Part model, mm, in its own coordinate system. Face numbers are marked on the shaded views. A direction names the side the tool comes from. Coordinates: 2 decimals unless noted, no trailing zeros. Loops run counter-clockwise (first coordinate to the right, second up) from the corner with the lowest first, then second, coordinate; pieces in that order, holes last. Notation, with made-up numbers: M 53.5,-14 L 108.5,-14 A20 cw 108.5,-10 Z; hole C 65,-33 d10. An arc over 180 degrees is marked long. Answer as a JSON object with one key per item and string values. Group by question number.
1. Mould opens along Z. For the marked faces 1, 2 and 3 say: released by +Z, released by -Z, zero draft, split by the parting line, or undercut.
2. Saw through at A-A on y = 0.3. Write the cut outline in (x, z) (3 decimals), then the cut area to 3 significant figures.
3. Drill centre lines: L1, parallel to Z at x = -1.25, y = 1.1 (3 decimals); L2, parallel to X at y = 0.4, z = 0.5 (3 decimals); L3, parallel to Z at x = -1.25, y = 3.05. Where is each one in solid material? Low to high.
4. Drop flat-ended pins along their axis: pin 1 Ø4 at (x, z) = (-4, -3) entering from -Y; pin 2 Ø0.6 at (x, y) = (-0.5, 0.5) entering from +Z. Give the stop position or say it passes through.
5. Saw through at B-B on x = -4. Write the cut outline in (y, z) (3 decimals).
6. Saw through at C-C on z = -4.25. Write the cut outline in (x, y) (3 decimals).
7. 3-axis set-ups, long thin cutter, end or side, ignore diameter. For the marked faces 4 and 5: which of +Z, -Z, +X, -X, +Y, -Y reach the whole face in a straight line?
Autodesk Inventor part; units mm, degrees
ref_plane "YZ Plane" through (0, 0, 0) normal (1, 0, 0) x (0, 1, 0)
ref_plane "XZ Plane" through (0, 0, 0) normal (0, 1, 0) x (-1, 0, 0)
ref_plane "XY Plane" through (0, 0, 0) normal (0, 0, 1) x (1, 0, 0)
sketch "Sketch1" plane through (0, 0, 0) normal (0, 1, 0) x (-1, 0, 0)
  circle A0 centre (0, 0) radius 0.36
  circle A1 centre (0, 0) radius 5
  dimension "d0" = 0.72
  dimension "d2" = 10
extrude "Extrusion1" add sketch "Sketch1" along normal blind 3.125
sketch "Sketch2" plane through (0, 3.125, 0) normal (0, 1, 0) x (1, 0, 0)
  circle A0 centre (0, 0) radius 1.5
  dimension "d10" = 3
sketch "Sketch3" plane through (0, 0, 0) normal (0, -1, 0) x (1, 0, 0)
  line L0 (-1.775, 1.775) -> (1.775, 1.775)
  line L1 (1.775, 1.775) -> (1.775, -1.775)
  line L2 (1.775, -1.775) -> (-1.775, -1.775)
  line L3 (-1.775, -1.775) -> (-1.775, 1.775)
  line L4 (-1.775, 1.775) -> (1.775, -1.775) construction
  line L5 (1.775, 1.775) -> (-1.775, -1.775) construction
  arc A0 (1.775, 1.475) -> (1.475, 1.775) centre (1.775, 1.775) ccw
  arc A1 (1.475, -1.775) -> (1.775, -1.475) centre (1.775, -1.775) ccw
  arc A2 (-1.775, -1.475) -> (-1.475, -1.775) centre (-1.775, -1.775) ccw
  arc A3 (-1.475, 1.775) -> (-1.775, 1.475) centre (-1.775, 1.775) ccw
  point P0 (0, 0)
  dimension "d11" = 0.3
  dimension "d13" = 3.55
extrude "Extrusion2" cut sketch "Sketch3" against normal blind 1.275
sketch "Sketch5" plane through (0, 0, 0) normal (0, 0, 1) x (1, 0, 0)
  line L0 (-0.36, 1.275) -> (0.36, 1.275)
  line L1 (5, 3.125) -> (-5, 3.125)
  arc A0 (-0.36, 1.275) -> (-1.5, 3.125) centre (-11.1041, -4.0695) ccw
  line L2 (0, 1.275) -> (0, 3.125)
  line L3 (0.36, 1.275) -> (0, 1.275)
  line L4 (0.36, 3.125) -> (0.36, 1.275)
  line L5 (0.36, 3.125) -> (-1.5, 3.125)
  point P0 (0, 0)
  dimension "d17" = 1.5
  dimension "d23" = 12
revolve "Revolution1" cut sketch "Sketch5" angle 360 about axis through (0, 1.275, 0) along (0, 1, 0) contours A0 L1 L2 L0
fillet "Fillet1" radius 0.05 1 edges at (0.36, 1.275, 0)
equation "\"d17\" = 0.5 * d10"
properties part number "Acoustic Horn 45deg V1"
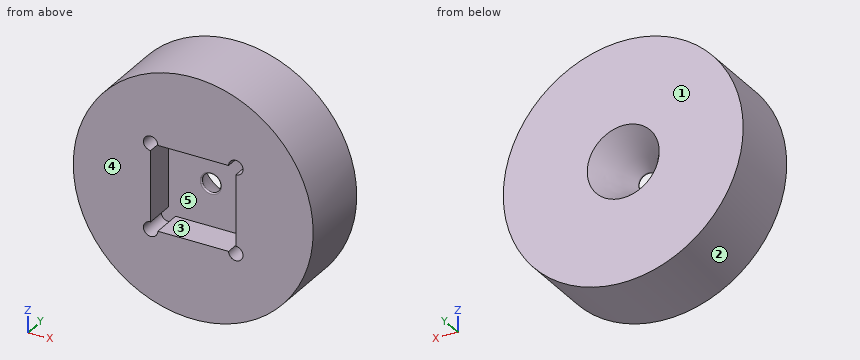
Outcome:
{
 "1": {"face 1": "zero draft", "face 2": "split by the parting line", "face 3": "undercut"},
 "2": {"outline": "C 0,0 d10; hole M -1.775,-1.475 A0.3 ccw long -1.475,-1.775 L 1.475,-1.775 A0.3 ccw long 1.775,-1.475 L 1.775,1.475 A0.3 ccw long 1.475,1.775 L -1.475,1.775 A0.3 ccw long -1.775,1.475 Z", "area": "65.1 mm²"},
 "3": {"L1": "z = -4.841 to -1.775, 1.775 to 4.841", "L2": "x = -4.975 to -1.775, 1.775 to 4.975", "L3": "z = -4.84 to -0.72, 0.72 to 4.84"},
 "4": {"pin 1": "stops at y = 0", "pin 2": "stops at z = 5"},
 "5": {"outline": "M 0,-3 L 3.125,-3 L 3.125,3 L 0,3 Z"},
 "6": {"outline": "M -2.634,0 L 2.634,0 L 2.634,3.125 L -2.634,3.125 Z"},
 "7": {"face 4": "+Z, -Z, +X, -X, -Y", "face 5": "-Y"}
}
